Check sheet for the modelled part. Datum: model origin and axes. Units: mm. A direction names the side the tool comes from. Coordinates: 2 decimals unless noted, no trailing zeros. Loops run counter-clockwise (first coordinate to the right, second up) from the corner with the lowest first, then second, coordinate; pieces in that order, holes last. Notation, with made-up numbers: M 3.5,55.25 L 56.5,55.25 A26 cw 56.5,88.25 Z; hole C 53,-35 d4. An arc over 180 degrees is marked long. Return JSON: item names as keys, results as strings.
from build123d import *

# Parameters (mm, degrees)
TROU_TARAUD_M8X1_01_D     = 7
TROU_TARAUD_M8X1_01_DEPTH = 30
TROU_TARAUD_M8X1_01_TIP   = 2.103012167
TROU_TARAUD_M41_REACH     = 58.745
TROU_TARAUD_M41_BORE_R    = 1.65
TROU_TARAUD_M42_REACH     = 58.745
TROU_TARAUD_M42_BORE_R    = 1.65


with BuildPart() as part:
    # Sketch1 → Revolve1 (revolve)
    with BuildSketch(Plane.XY, mode=Mode.PRIVATE) as revolve1_sk:
        Polygon((-5, 12), (-5, 7), (0, 7), (0, 0), (-50, 0), (-50, 7), (-12, 7), (-12, 12), align=None)
    revolve(revolve1_sk.sketch.rotate(Axis((-78.343949045, 0, 0), (1, 0, 0)), 90), axis=Axis((-78.343949045, 0, 0), (1, 0, 0)))

    # Trou taraudé M8x1.01
    with Locations(Plane(origin=(0, 0, 0), x_dir=(0, 0, -1), z_dir=(1, 0, 0))):
        with Locations((0, 0)):
            Hole(TROU_TARAUD_M8X1_01_D / 2, depth=TROU_TARAUD_M8X1_01_DEPTH)
            with Locations((0, 0, -(TROU_TARAUD_M8X1_01_DEPTH + TROU_TARAUD_M8X1_01_TIP / 2))):  # 118° drill point
                Cone(0, TROU_TARAUD_M8X1_01_D / 2, TROU_TARAUD_M8X1_01_TIP, mode=Mode.SUBTRACT)

    # Trou taraudé M41 bore → Trou taraudé M41 (cut, up to next)
    with BuildSketch(Plane.XY.offset(12), mode=Mode.PRIVATE) as trou_taraud_m41_sk1:
        with Locations((-8.5, 0)):
            Circle(TROU_TARAUD_M41_BORE_R)
    trou_taraud_m41_tool1 = extrude(trou_taraud_m41_sk1.sketch, amount=-TROU_TARAUD_M41_REACH, mode=Mode.PRIVATE) & part.part
    add(trou_taraud_m41_tool1.solids().sort_by_distance((-8.5, 0, 12))[0], mode=Mode.SUBTRACT)

    # Trou taraudé M42 bore → Trou taraudé M42 (cut, up to next)
    with BuildSketch(Plane(origin=(0, 12, 0), x_dir=(1, 0, 0), z_dir=(0, 1, 0)), mode=Mode.PRIVATE) as trou_taraud_m42_sk1:
        with Locations((-8.5, 0)):
            Circle(TROU_TARAUD_M42_BORE_R)
    trou_taraud_m42_tool1 = extrude(trou_taraud_m42_sk1.sketch, amount=-TROU_TARAUD_M42_REACH, mode=Mode.PRIVATE) & part.part
    add(trou_taraud_m42_tool1.solids().sort_by_distance((-8.5, 12, 0))[0], mode=Mode.SUBTRACT)


solid = part.part
1) Section check D-D on y = 10.5. Record the cut outline in (x, z).
Answers:
{"outline": "M -12,-5.81 L -5,-5.81 L -5,5.81 L -12,5.81 Z; hole C -8.5,0 d3.3"}
2) Draft check along Z on faces 5 (the face through (-8.451, -3.604, 11.446)), 6 (the face through (0, 3, 3)), 7 (the face through (-15.2, -2.1, -2.8)). Enter one of: +Z half, -Z half, draft (parallel to the pull), parting line (faces both ways), or undercut.
Answers:
{"face 5": "parting line", "face 6": "draft", "face 7": "undercut"}
3) Section check B-B on x = -8.5. Record the cut outline in (y, z).
Answers:
{"outline": "M -1.65,3.09 L -1.65,11.89 A12 ccw long 11.89,-1.65 L 3.09,-1.65 A3.5 cw long Z; M 1.65,3.09 A3.5 cw 3.09,1.65 L 11.89,1.65 A12 ccw 1.65,11.89 Z"}
4) Section check C-C on x = -18. Record the cut outline in (y, z).
Answers:
{"outline": "C 0,0 d14; hole C 0,0 d7"}
5) Go/stop test with flat-tipped pins: pin 1 Ø6 at (y, z) = (-5, 9.5) entering from -X; pin 2 Ø1 at (y, z) = (-7.5, -2) entering from +X; pin 3 Ø5 at (x, y) = (-34, -3.5) entering from -Z. Record where each tip stops, or that it passes through.
Answers:
{"pin 1": "x = -12", "pin 2": "x = -5", "pin 3": "z = -6.93"}
6) Scan lines: line 1 along X through (y, z) = (10, 0); line 2 along Y through (x, z) = (-16.5, 0); line 3 along Z through (x, y) = (-7.5, 3.5). Record each from-to range of solid material in increasing order. Write a range as [from, to].
Answers:
{"line 1": "[-12, -10.15], [-6.85, -5]", "line 2": "[-7, -3.5], [3.5, 7]", "line 3": "[-11.48, -1.31], [1.31, 11.48]"}
7) Set-up check for faces 1 (the face through (-5, 5.2, 5.2)), 2 (the face through (-12, 5.2, -5.2)), 3 (the face through (-10.15, 0.07, 7.61)), 4 (the face through (-9.81, 7.61, 1)): record each of +Z, -Z, +X, -X, +Y, -Y from which the full face is reachable in a straight line by a thin tool's end or side.
Answers:
{"face 1": "+X", "face 2": "-X", "face 3": "+Z", "face 4": "+Y"}
8) Section check A-A on z = 10.25. Record the cut outline in (x, y), then the cut area to 3 significant figures.
Answers:
{"outline": "M -12,-6.24 L -5,-6.24 L -5,6.24 L -12,6.24 Z; hole C -8.5,0 d3.3", "area": "78.8 mm²"}
